```python
from build123d import *

# Parameters (mm, degrees)
BOSS_EXTRUDE1_DEPTH                              = 5
CSK_FOR_8_FLAT_HEAD_SOCKET_CAP_SCREW1_A_COUNT    = 2
CSK_FOR_8_FLAT_HEAD_SOCKET_CAP_SCREW1_A_PITCH    = 75
CSK_FOR_8_FLAT_HEAD_SOCKET_CAP_SCRE_2_COUNT      = 2
CSK_FOR_8_FLAT_HEAD_SOCKET_CAP_SCRE_2_PITCH      = 116.215709833
CSK_FOR_8_FLAT_HEAD_SOCKET_CAP_SCRE_3_COUNT      = 2
CSK_FOR_8_FLAT_HEAD_SOCKET_CAP_SCRE_3_PITCH      = 88.775510204
CSK_FOR_8_FLAT_HEAD_SOCKET_CAP_SCRE_4_COUNT      = 2
CSK_FOR_8_FLAT_HEAD_SOCKET_CAP_SCRE_4_PITCH      = 58.107854917
SKETCH4_R                                        = 5
BOSS_EXTRUDE2_DEPTH                              = 5
CHAMFER1_SIZE                                    = 2
CBORE_FOR_M5_HEX_HEAD_MACHINE_SCREW1_D           = 4.25
CBORE_FOR_M5_HEX_HEAD_MACHINE_SCREW1_CBORE_D     = 5
CBORE_FOR_M5_HEX_HEAD_MACHINE_SCREW1_CBORE_DEPTH = 0.5


with BuildPart() as part:
    # Sketch1 → Boss-Extrude1 (new body)
    with BuildSketch(Plane(origin=(0, 0, 0), x_dir=(1, 0, 0), z_dir=(0, 1, 0))):
        with BuildLine():
            Line((0, -11.621570983), (-9.818223762, 0))
            Line((-9.818223762, 0), (-43.229142192, -39.547617733))
            ThreePointArc((-43.229142192, -39.547617733), (-42.340137369, -50.116897294), (-31.770857808, -49.227892471))
            Line((-31.770857808, -49.227892471), (0, -11.621570983))
        make_face()
        Polygon((9.818223762, 0), (0, 11.621570983), (-9.818223762, 0), (0, -11.621570983), align=None)
        with BuildLine():
            Line((0, 11.621570983), (-31.770857808, 49.227892471))
            ThreePointArc((-31.770857808, 49.227892471), (-42.340137369, 50.116897294), (-43.229142192, 39.547617733))
            Line((-43.229142192, 39.547617733), (-9.818223762, 0))
            Line((-9.818223762, 0), (0, 11.621570983))
        make_face()
        with BuildLine():
            Line((31.770857808, 49.227892471), (0, 11.621570983))
            Line((0, 11.621570983), (9.818223762, 0))
            Line((9.818223762, 0), (43.229142192, 39.547617733))
            ThreePointArc((43.229142192, 39.547617733), (42.340137369, 50.116897294), (31.770857808, 49.227892471))
        make_face()
        with BuildLine():
            Line((43.229142192, -39.547617733), (9.818223762, 0))
            Line((9.818223762, 0), (0, -11.621570983))
            Line((0, -11.621570983), (31.770857808, -49.227892471))
            ThreePointArc((31.770857808, -49.227892471), (42.340137369, -50.116897294), (43.229142192, -39.547617733))
        make_face()
    extrude(amount=BOSS_EXTRUDE1_DEPTH)

    # Sketch3 → CSK for #8 Flat Head Socket Cap Screw1 (revolve, cut)
    with BuildSketch(Plane(origin=(-37.5, 5, -44.387755102), x_dir=(0, 0, 1), z_dir=(1, 0, 0))):
        Polygon((0, 0), (0, 5), (2.2479, 5), (2.2479, 3.257958366), (5.08, 0), align=None)
    csk_for_8_flat_head_socket_cap_screw1 = revolve(axis=Axis((-37.5, 11.35, -44.387755102), (0, -1, 0)), mode=Mode.SUBTRACT)

    # CSK for #8 Flat Head Socket Cap Screw1 a: CSK for #8 Flat Head Socket Cap Screw1 ×2
    with Locations(*[(i * CSK_FOR_8_FLAT_HEAD_SOCKET_CAP_SCREW1_A_PITCH, 0, 0) for i in range(1, CSK_FOR_8_FLAT_HEAD_SOCKET_CAP_SCREW1_A_COUNT)]):
        add(csk_for_8_flat_head_socket_cap_screw1, mode=Mode.SUBTRACT)

    # CSK for _8 Flat Head Socket Cap Scre 2: CSK for #8 Flat Head Socket Cap Screw1 ×2
    with Locations(*[Vector(0.6453516491682099, 0, 0.7638856255460446) * (i * CSK_FOR_8_FLAT_HEAD_SOCKET_CAP_SCRE_2_PITCH) for i in range(1, CSK_FOR_8_FLAT_HEAD_SOCKET_CAP_SCRE_2_COUNT)]):
        add(csk_for_8_flat_head_socket_cap_screw1, mode=Mode.SUBTRACT)

    # CSK for _8 Flat Head Socket Cap Scre 3: CSK for #8 Flat Head Socket Cap Screw1 ×2
    with Locations(*[(0, 0, i * CSK_FOR_8_FLAT_HEAD_SOCKET_CAP_SCRE_3_PITCH) for i in range(1, CSK_FOR_8_FLAT_HEAD_SOCKET_CAP_SCRE_3_COUNT)]):
        add(csk_for_8_flat_head_socket_cap_screw1, mode=Mode.SUBTRACT)

    # CSK for _8 Flat Head Socket Cap Scre 4: CSK for #8 Flat Head Socket Cap Screw1 ×2
    with Locations(*[Vector(0.64535164916821, 0, 0.7638856255460446) * (i * CSK_FOR_8_FLAT_HEAD_SOCKET_CAP_SCRE_4_PITCH) for i in range(1, CSK_FOR_8_FLAT_HEAD_SOCKET_CAP_SCRE_4_COUNT)]):
        add(csk_for_8_flat_head_socket_cap_screw1, mode=Mode.SUBTRACT)

    # Sketch4 → Boss-Extrude2 (add)
    with BuildSketch(Plane(origin=(0, 5, 0), x_dir=(1, 0, 0), z_dir=(0, 1, 0))):
        with Locations(Location((-24.5, 29, 0), (0, 0, 270))):
            Circle(SKETCH4_R)
        with Locations(Location((24.5, 29, 0), (0, 0, 270))):
            Circle(SKETCH4_R)
        with Locations(Location((24.5, -29, 0), (0, 0, 270))):
            Circle(SKETCH4_R)
        with Locations(Location((-24.5, -29, 0), (0, 0, 270))):
            Circle(SKETCH4_R)
    extrude(amount=BOSS_EXTRUDE2_DEPTH)

    # Chamfer1
    chamfer1_edges = [part.edges().sort_by_distance(p)[0] for p in [
        (-24.5, 5, -34),
        (24.5, 5, -34),
        (24.5, 5, 24),
        (-24.5, 5, 24),
    ]]
    chamfer(chamfer1_edges, length=CHAMFER1_SIZE)

    # CBORE for M5 Hex Head Machine Screw1 (through all)
    with Locations(Plane(origin=(0, 10, 0), x_dir=(1, 0, 0), z_dir=(0, 1, 0))):
        with Locations((-24.5, 29), (24.5, 29), (24.5, -29), (-24.5, -29)):
            CounterBoreHole(CBORE_FOR_M5_HEX_HEAD_MACHINE_SCREW1_D / 2, CBORE_FOR_M5_HEX_HEAD_MACHINE_SCREW1_CBORE_D / 2, CBORE_FOR_M5_HEX_HEAD_MACHINE_SCREW1_CBORE_DEPTH)

    # Fillet1
    # a fillet whose section is not a circle: 20 mm, written as the material it adds along each edge
    with BuildSketch(Plane(origin=(-9.818223762, 0, 0), x_dir=(-0.6453516491682094, 0, 0.7638856255460448), z_dir=(0, 1, 0))) as fillet1_piece_1:
        with BuildLine():
            Bezier((16.896551724, 0), (0, 0), (-2.822442205, -16.659150043), weights=[1, 1.5, 1])
            Line((-2.822442205, -16.659150043), (0, 0))
            Line((0, 0), (16.896551724, 0))
        make_face()
    extrude(amount=5)
    with BuildSketch(Plane(origin=(9.818223762, 0, 0), x_dir=(0.6453516491682099, 0, 0.7638856255460446), z_dir=(0, 1, 0))) as fillet1_piece_2:
        with BuildLine():
            Bezier((16.896551724, 0), (0, 0), (-2.822442205, 16.659150043), weights=[1, 1.5, 1])
            Line((-2.822442205, 16.659150043), (0, 0))
            Line((0, 0), (16.896551724, 0))
        make_face()
    extrude(amount=5)
    with BuildSketch(Plane(origin=(0, 0, 11.621570983), x_dir=(-0.6453516491682095, 0, 0.7638856255460447), z_dir=(0, 1, 0))) as fillet1_piece_3:
        with BuildLine():
            Bezier((23.673469388, 0), (0, 0), (3.954475459, 23.340849957), weights=[1, 1.5, 1])
            Line((3.954475459, 23.340849957), (0, 0))
            Line((0, 0), (23.673469388, 0))
        make_face()
    extrude(amount=5)
    with BuildSketch(Plane(origin=(0, 0, -11.621570983), x_dir=(-0.6453516491682103, 0, -0.7638856255460442), z_dir=(0, 1, 0))) as fillet1_piece_4:
        with BuildLine():
            Bezier((23.673469388, 0), (0, 0), (3.954475459, -23.340849957), weights=[1, 1.5, 1])
            Line((3.954475459, -23.340849957), (0, 0))
            Line((0, 0), (23.673469388, 0))
        make_face()
    extrude(amount=5)


solid = part.part
```
The listing builds one solid part. Answer for the finished solid, in the listing's coordinates (mm). A direction names the side the tool comes from. Give positions to 0.01 mm unless a question says otherwise; leave off trailing zeros. Order: outer loops, then holes, each group sorted by start corner. A loop starts at its lowest first (then second) coordinate and runs counter-clockwise, first axis right, second up. Notation, with made-up numbers: (61.25, 13) -> (73.25, 13) arc R23 ccw to (73.25, 21) -> close; hole circle Ø7 at (47.25, 37.25). An arc over 180 degrees is marked (long way). One line per item, written item: value.
1) Find section B-B, the plane z = -37.5. Determine the outline of the cut face in (x, y), plus the area to 3 significant figures.
Reported:
outline: (-41.5, 0) -> (-21.86, 0) -> (-21.86, 5) -> (-41.5, 5) -> close; (21.86, 0) -> (41.5, 0) -> (41.5, 5) -> (21.86, 5) -> close
area: 196 mm^2
2) Find section A-A, the plane x = 37.5. Determine the outline of the cut face in (y, z), plus the area to 3 significant figures.
Reported:
outline: (0, -51.89) -> (5, -51.89) -> (5, -49.47) -> (1.74, -46.64) -> (0, -46.64) -> close; (0, -42.14) -> (1.74, -42.14) -> (5, -39.31) -> (5, -32.77) -> (0, -32.77) -> close; (0, 32.77) -> (5, 32.77) -> (5, 39.31) -> (1.74, 42.14) -> (0, 42.14) -> close; (0, 46.64) -> (1.74, 46.64) -> (5, 49.47) -> (5, 51.89) -> (0, 51.89) -> close
area: 128 mm^2
3) Find section C-C, the plane y = 3.5. Count the separate pieces of the cut face and the enclosed holes in it, plus the area to 3 significant figures.
Reported:
separate pieces: 1
enclosed holes: 9
area: 3,530 mm^2
4) Determine the mould class of faces 1 (the flat face through (23.41, 2.46, 39.33)), 2 (the flat face through (-22, 10, 30)), 3 (the flat face through (-23.41, 2.46, -39.33)), 4 (the cylindrical face through (-22.81, 4.68, 30.29)) for opening direction Z: pulls with the +Z half, pulls with the -Z half, needs draft (parallel to the pull), parting line crosses it, or undercut.
Reported:
face 1: pulls with the +Z half
face 2: needs draft
face 3: pulls with the -Z half
face 4: undercut
5) A tool of negligible diameter and unlimited length cuts with its end or side. For faces 5 (the flat face through (27, 10, -28)), 6 (the flat face through (-31.82, 2.46, 26.04)), 7 (the cylindrical face through (-27.5, 8.5, 25)), 8 (the flat face through (31.82, 2.46, -26.04)), 9 (the flat face through (23.64, 2.465, -39.603)), from which of +Z, -Z, +X, -X, +Y, -Y can it reach the whole face along a straight path? Write none if from no direction.
Reported:
face 5: +Z, -Z, +X, -X, +Y
face 6: -X, +Y, -Y
face 7: +Y
face 8: +X, +Y, -Y
face 9: -Z, +Y, -Y
6) Find section D-D, the plane z = -16. Determine the outline of the cut face in (x, y).
Reported:
outline: (-23.34, 0) -> (23.34, 0) -> (23.34, 5) -> (-23.34, 5) -> close
7) Find the intervals of material crossed by line 1 (X direction, y = 2, z = 29) (3 decimals); line 2 (Z direction, x = 23, y = 7.5); line 3 (Z direction, x = 24.5, y = 6) (3 decimals), in increasing order.
Reported:
line 1: x = -34.318 to -26.625, -22.375 to -14.676, 14.676 to 22.375, 26.625 to 34.318
line 2: z = -33.77 to -30.51, -27.49 to -24.23, 24.23 to 27.49, 30.51 to 33.77
line 3: z = -35 to -31.125, -26.875 to -23, 23 to 26.875, 31.125 to 35
8) Flat-ended cylindrical pins translate along their axes: P1, Ø1.5, axis at y = 2.5, z = 35, coming from the -X side; P2, Ø6, axis at x = 20.5, y = 2.5, coming from the -Z side; P3, Ø1.5, axis at x = -10.5, z = -8.5, coming from the +Y side. Find the tip coordinate at first contact, or state that the pin passes through.
Reported:
P1: stops at x = -40.02
P2: stops at z = -39.44
P3: stops at y = 5
